Work out the finished part from the listing and answer in its coordinate system (mm). Round coordinates to 2 decimals unless told otherwise and drop trailing zeros. Loops run counter-clockwise (first coordinate to the right, second up) from the corner with the lowest first, then second, coordinate; pieces in that order, holes last. Notation, with made-up numbers: (66.5, 52) -> (91.5, 52) arc R16 ccw to (91.5, 62) -> close; hole circle Ø5 at (16.5, 82.25). An arc over 180 degrees is marked (long way). Use one line per item in the form item = value.
```python
from build123d import *

# Parameters (mm, degrees)
SKETCH1_R           = 1.4224
BOSS_EXTRUDE7_DEPTH = 2.9718


with BuildPart() as part:
    # Sketch1 → Boss-Extrude7 (new body)
    with BuildSketch(Plane.XY):
        Polygon((15.494, 22.4282), (2.9718, 22.4282), (2.9718, 16.256), (0, 16.256), (0, 9.144), (2.9718, 9.144), (2.9718, 0), (0, 0), (0, -4.445), (16.51, -5.08), (0, -5.715), (0, -8.255), (16.51, -8.89), (0, -9.525), (0, -12.065), (16.51, -12.7), (0, -13.335), (0, -15.875), (16.51, -16.51), (0, -17.145), (0, -19.685), (16.51, -20.32), (0, -20.955), (0, -25.4), (38.1, -25.4), (38.1, -20.955), (21.59, -20.32), (38.1, -19.685), (38.1, -17.145), (21.59, -16.51), (38.1, -15.875), (38.1, -13.335), (21.59, -12.7), (38.1, -12.065), (38.1, -9.525), (21.59, -8.89), (38.1, -8.255), (38.1, -5.715), (21.59, -5.08), (38.1, -4.445), (38.1, 22.4282), (22.606, 22.4282), (22.606, 25.4), (15.494, 25.4), align=None)
        with Locations((1.4859, 12.7)):
            Circle(SKETCH1_R, mode=Mode.SUBTRACT)
        with Locations((19.05, 23.9141)):
            Circle(SKETCH1_R, mode=Mode.SUBTRACT)
        Polygon((2.54, -6.985), (19.05, -6.35), (35.56, -6.985), (19.05, -7.62), align=None, mode=Mode.SUBTRACT)
        Polygon((19.05, -19.05), (2.54, -18.415), (19.05, -17.78), (35.56, -18.415), align=None, mode=Mode.SUBTRACT)
        Polygon((19.05, -13.97), (35.56, -14.605), (19.05, -15.24), (2.54, -14.605), align=None, mode=Mode.SUBTRACT)
        Polygon((19.05, -10.16), (35.56, -10.795), (19.05, -11.43), (2.54, -10.795), align=None, mode=Mode.SUBTRACT)
    extrude(amount=BOSS_EXTRUDE7_DEPTH)


solid = part.part
```
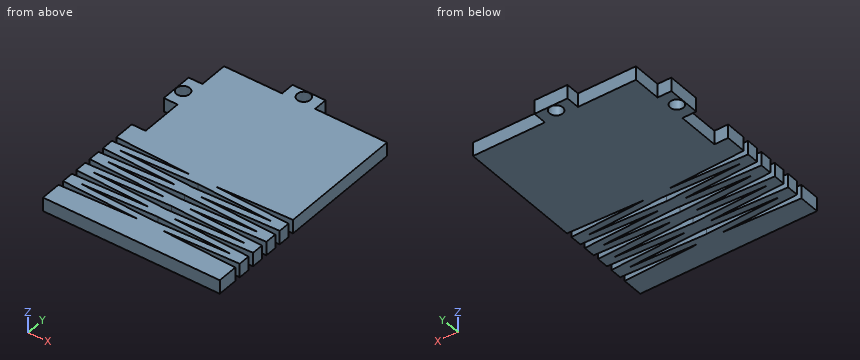
(1) Find section B-B, the plane x = 8.5. State how many separate pieces and enclosed holes the cut face has, then the cut area to 3 significant figures.
Completed:
separate_pieces = 10
enclosed_holes = 0
area = 128 mm2
(2) Consider L1, parallel to X at y = 6, z = 0.35. Determine where the line is inside the solid, lowest interval first.
Completed:
L1 = 2.97 to 38.1
(3) Given P1, Ø1.5, axis at x = 8, z = 2, coming from the +Y side; P2, Ø0.9, axis at y = 23.5, z = 1.5, coming from the +X side; P3, Ø1.7, axis at x = 1.49, y = 12.7, coming from the -Z side; P4, Ø1.5, axis at x = 1, z = 2, coming from the +Y side, each flat-ended and moving along its own axis, determine where each tip first touches the part or whether it passes through.
Completed:
P1 = 22.43
P2 = 22.61
P3 = through
P4 = 16.26
(4) Find section A-A, the plane y = 12.7. Write down the section's boundary in (x, z), then the cut area to 3 significant figures.
Completed:
outline = (0, 0) -> (0.06, 0) -> (0.06, 2.97) -> (0, 2.97) -> close; (2.91, 0) -> (38.1, 0) -> (38.1, 2.97) -> (2.91, 2.97) -> close
area = 105 mm2
